```python
from build123d import *

# Parameters (mm, degrees)
SKETCH_1_R      = 14
EXTRUDE_1_DEPTH = 12
SKETCH_2_R      = 11
EXTRUDE_2_DEPTH = 3
SKETCH_3_R      = 18
EXTRUDE_3_DEPTH = 10
SKETCH_4_W      = 30
SKETCH_4_H      = 33
EXTRUDE_4_DEPTH = 40


with BuildPart() as part:
    # 草图1 → 凸台-拉伸1 (new body)
    with BuildSketch(Plane.XY):
        Circle(SKETCH_1_R)
    extrude(amount=EXTRUDE_1_DEPTH)

    # 草图2 → 凸台-拉伸2 (add)
    with BuildSketch(Plane(origin=(0, 0, 0), x_dir=(-1, 0, 0), z_dir=(0, 0, -1))):
        Circle(SKETCH_2_R)
    extrude(amount=EXTRUDE_2_DEPTH)

    # 草图3 → 凸台-拉伸3 (add)
    with BuildSketch(Plane(origin=(0, 0, -3), x_dir=(-1, 0, 0), z_dir=(0, 0, -1))):
        Circle(SKETCH_3_R)
    extrude(amount=EXTRUDE_3_DEPTH)

    # 草图4 → 凸台-拉伸4 (add)
    with BuildSketch(Plane(origin=(0, 0, -13), x_dir=(-1, 0, 0), z_dir=(0, 0, -1))):
        Rectangle(SKETCH_4_W, SKETCH_4_H)
    extrude(amount=EXTRUDE_4_DEPTH)


solid = part.part
```
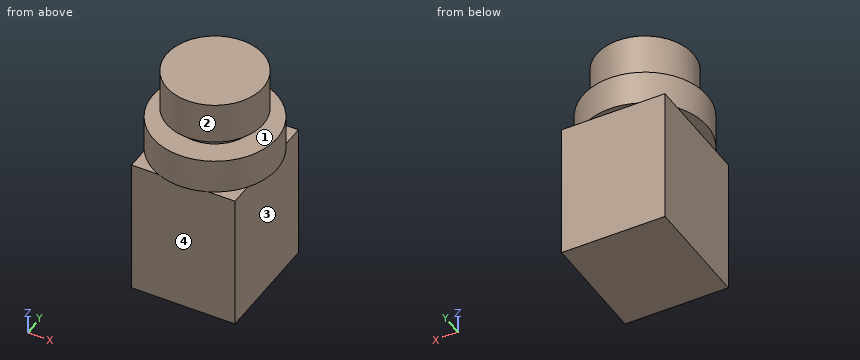
Geometry check sheet. Reference: the model listing, model coordinates, mm. Face numbers are marked on the shaded views. A direction names the side the tool comes from. Round coordinates to 2 decimals unless told otherwise and drop trailing zeros. Loops run counter-clockwise (first coordinate to the right, second up) from the corner with the lowest first, then second, coordinate; pieces in that order, holes last. Notation, with made-up numbers: (21, 33) - (54, 33) arc R19 cw to (54, 51) - close; hole circle Ø1 at (60.25, 11). An arc over 180 degrees is marked (long way). Use a Markdown table: item, result.
Q1. Go/stop test with flat-tipped pins: P1, Ø7, axis at x = -12, y = 14, coming from the +Z side; P2, Ø8, axis at y = -3.5, z = -16, coming from the +X side; P3, Ø2.5, axis at x = 17, y = 4, coming from the -Z side. Record where each tip stops, or that it passes through.
Solutions:
| item | result |
|---|---|
| P1 | stops at z = -3 |
| P2 | stops at x = 17.98 |
| P3 | stops at z = -13 |
Q2. Material ranges on line 1 (Z direction, x = 1, y = -13.5); line 2 (X direction, y = 6.5, z = -35); line 3 (Y direction, x = 11, z = -24), recorded low to high.
Solutions:
| item | result |
|---|---|
| line 1 | z = -53 to -3, 0 to 12 |
| line 2 | x = -15 to 15 |
| line 3 | y = -16.5 to 16.5 |
Q3. Cross-section at A-A on x = 0. Record the cut outline in (y, z), plus the area to 3 significant figures.
Solutions:
| item | result |
|---|---|
| outline | (-18, -13) - (-16.5, -13) - (-16.5, -53) - (16.5, -53) - (16.5, -13) - (18, -13) - (18, -3) - (11, -3) - (11, 0) - (14, 0) - (14, 12) - (-14, 12) - (-14, 0) - (-11, 0) - (-11, -3) - (-18, -3) - close |
| area | 2,080 mm2 |
Q4. Cross-section at B-B on y = 0. Record the cut outline in (x, z).
Solutions:
| item | result |
|---|---|
| outline | (-18, -13) - (-15, -13) - (-15, -53) - (15, -53) - (15, -13) - (18, -13) - (18, -3) - (11, -3) - (11, 0) - (14, 0) - (14, 12) - (-14, 12) - (-14, 0) - (-11, 0) - (-11, -3) - (-18, -3) - close |
Q5. Cross-section at D-D on x = -13. Record the cut outline in (y, z), plus the area to 3 significant figures.
Solutions:
| item | result |
|---|---|
| outline | (-16.5, -53) - (16.5, -53) - (16.5, -13) - (12.45, -13) - (12.45, -3) - (-12.45, -3) - (-12.45, -13) - (-16.5, -13) - close; (-5.2, 0) - (5.2, 0) - (5.2, 12) - (-5.2, 12) - close |
| area | 1,690 mm2 |
Q6. Cross-section at C-C on z = -32.5. Record the cut outline in (x, y), plus the area to 3 significant figures.
Solutions:
| item | result |
|---|---|
| outline | (-15, -16.5) - (15, -16.5) - (15, 16.5) - (-15, 16.5) - close |
| area | 990 mm2 |
Q7. Access from +Z, -Z, +X, -X, +Y, -Y to the whole of each face (thin tool, end or side, straight path). Record for the marked faces 1, 2, 3 and 4.
Solutions:
| item | result |
|---|---|
| face 1 | none |
| face 2 | +Z |
| face 3 | -Z, +X, +Y, -Y |
| face 4 | -Z, +X, -X, -Y |
